For this review, take the finished solid that the model builds, in its own axes (mm). A direction names the side the tool comes from. Coordinates: 2 decimals unless noted, no trailing zeros. Loops run counter-clockwise (first coordinate to the right, second up) from the corner with the lowest first, then second, coordinate; pieces in that order, holes last. Notation, with made-up numbers: M 84.5,47 L 139.5,47 A17 cw 139.5,54 Z; hole C -28.5,85 d4. An arc over 180 degrees is marked long. Write item = value, one per line.
from build123d import *

# Parameters (mm, degrees)
SKETCH1_R           = 3.175
BOSS_EXTRUDE1_DEPTH = 25.4
CUT_EXTRUDE1_START  = -25.4
SKETCH2_W           = 12.7
SKETCH2_H           = 12.7
CUT_EXTRUDE1_DEPTH  = 1.5875
FILLET1_R           = 1.5875


with BuildPart() as part:
    # Sketch1 → Boss-Extrude1 (new body)
    with BuildSketch(Plane.XY):
        with BuildLine():
            Line((-25.4, 3.175), (-9.525, 3.175))
            Line((-9.525, 3.175), (-9.525, -6.35))
            Line((-9.525, -6.35), (0, -6.35))
            ThreePointArc((0, -6.35), (6.35, 0), (0, 6.35))
            Line((0, 6.35), (-25.4, 6.35))
            Line((-25.4, 6.35), (-25.4, 3.175))
        make_face()
        Circle(SKETCH1_R, mode=Mode.SUBTRACT)
    extrude(amount=BOSS_EXTRUDE1_DEPTH)

    # Sketch2 → Cut-Extrude1 (cut)
    with BuildSketch(Plane.XY.offset(25.4).offset(CUT_EXTRUDE1_START)):
        Rectangle(SKETCH2_W, SKETCH2_H)
    extrude(amount=CUT_EXTRUDE1_DEPTH, mode=Mode.SUBTRACT)

    # Fillet1
    fillet1_edges = [part.edges().sort_by_distance(p)[0] for p in [
        (-9.525, -6.35, 12.7),
        (-9.525, 3.175, 12.7),
        (-25.4, 6.35, 12.7),
        (-25.4, 3.175, 12.7),
    ]]
    fillet(fillet1_edges, radius=FILLET1_R - 0.0001)  # a hair under: the kernel refuses the full size


solid = part.part
Q1. For line 1 along X through (y, z) = (0, 20) (3 decimals); line 2 along Z through (x, y) = (3.5, -0.25); line 3 along X through (y, z) = (1.25, 3.75) (3 decimals), list the stretches that pass through material, from the lowest coordinate up.
Solved:
line_1 = -9.525 to -3.175, 3.175 to 6.35
line_2 = 1.59 to 25.4
line_3 = -9.525 to -2.919, 2.919 to 6.226
Q2. For pin 1 Ø5 at (x, y) = (-3.5, 0) entering from -Z; pin 2 Ø8 at (x, z) = (-20.5, 6) entering from -Y (3 decimals); pin 3 Ø1 at (y, z) = (3, 6) entering from -X (3 decimals); pin 4 Ø5 at (x, y) = (0, 0) entering from -Z, all flat-tipped, find the tip position at first contact; note any pin that passes through.
Solved:
pin_1 = 1.59
pin_2 = 3.175
pin_3 = -24.775
pin_4 = through
Q3. Machinability: for faces 5 (the face through (-6.35, 0, 1)), 6 (the face through (-4, -6.35, 13)), which of the approach directions +Z, -Z, +X, -X, +Y, -Y give a long, thin tool a straight path to every point of the face, cutting with its end or side? Answer none if there is none.
Solved:
face_5 = -Z, +X, +Y, -Y
face_6 = +Z, -Z, +X, -X, -Y
Q4. Add section D-D (x = -23). Write out the cut boundary in (y, z) (3 decimals).
Solved:
outline = M 3.175,0 L 6.35,0 L 6.35,25.4 L 3.175,25.4 Z
Q5. Add section C-C (x = 1). Write out the cut boundary in (y, z), and give its area (3 significant figures).
Solved:
outline = M -6.27,1.59 L -3.01,1.59 L -3.01,25.4 L -6.27,25.4 Z; M 3.01,1.59 L 6.27,1.59 L 6.27,25.4 L 3.01,25.4 Z
area = 155 mm²
Q6. Draft analysis for pull direction Y (two halves, no side actions). For faces 1 (the face through (-9.525, -2, 13)), 2 (the face through (6.35, -0.14, 13.33)), 3 (the face through (-0.69, -3.1, 13.33)), 4 (the face through (-18, 3.175, 13)), state which applies: +Y half, -Y half, draft (parallel to the pull), parting line (faces both ways), or undercut.
Solved:
face_1 = draft
face_2 = parting line
face_3 = undercut
face_4 = -Y half
